```python
from build123d import *

# Parameters (mm, degrees)
SKETCH1_W           = 12.7
SKETCH1_H           = 31.75
SKETCH1_R           = 1.5875
BOSS_EXTRUDE2_DEPTH = 6.35
SKETCH1_5_R         = 1.27
CUT_EXTRUDE2_DEPTH  = 19.238986403
FILLET2_R           = 3.175
FILLET3_R           = 0.635


with BuildPart() as part:
    # Sketch1 → Boss-Extrude2 (new body)
    with BuildSketch(Plane(origin=(0, 0, 0), x_dir=(1, 0, 0), z_dir=(0, 1, 0))):
        Rectangle(SKETCH1_W, SKETCH1_H)
        with Locations(Location((0, -7.9375, 0), (0, 0, 270))):
            Circle(SKETCH1_R, mode=Mode.SUBTRACT)
    extrude(amount=BOSS_EXTRUDE2_DEPTH)

    # Sketch1_5 → Cut-Extrude2 (cut, through all)
    with BuildSketch(Plane(origin=(0, 0, 0), x_dir=(1, 0, 0), z_dir=(0, 1, 0))):
        with BuildLine():
            Line((-6.35, 3.701051224), (-6.35, -1.213547665))
            Line((-6.35, -1.213547665), (0.969401523, 7.434536298))
            ThreePointArc((0.969401523, 7.434536298), (-0.859985471, 7.320481413), (-0.898025612, 9.153025612))
            Line((-0.898025612, 9.153025612), (-6.35, 3.701051224))
        make_face()
        with Locations((0, 8.255)):
            Circle(SKETCH1_5_R)
    extrude(amount=CUT_EXTRUDE2_DEPTH, mode=Mode.SUBTRACT)

    # Fillet2
    fillet2_edges = [part.edges().sort_by_distance(p)[0] for p in [
        (6.35, 3.175, -15.875),
        (-6.35, 3.175, -15.875),
        (-6.35, 3.175, 15.875),
        (6.35, 3.175, 15.875),
    ]]
    fillet(fillet2_edges, radius=FILLET2_R)

    # Fillet3
    fillet3_edges = [part.edges().sort_by_distance(p)[0] for p in [
        (-6.35, 3.175, 1.213547665),
        (-6.35, 3.175, -3.701051224),
    ]]
    fillet(fillet3_edges, radius=FILLET3_R)


solid = part.part
```
Work out the finished part from the listing and answer in its coordinate system (mm). A direction names the side the tool comes from. Give positions to 0.01 mm unless a question says otherwise; leave off trailing zeros. Loops run counter-clockwise (first coordinate to the right, second up) from the corner with the lowest first, then second, coordinate; pieces in that order, holes last. Notation, with made-up numbers: (68.25, 86.25) -> (112.25, 86.25) arc R35 cw to (112.25, 122.25) -> close; hole circle Ø7 at (14, 30). An arc over 180 degrees is marked (long way). One line per question, with ' | ' between items. Start each with the question number.
1) Section B-B, the plane x = 0 is taken. Determine the outline of the cut face in (y, z) (3 decimals).
2) Section D-D, the plane x = 5 is taken. Determine the outline of the cut face in (y, z).
3) Determine the mould class of faces 3 (the face through (5.395, 3.219, -14.97)), 4 (the face through (-6.35, 3, 7)), 5 (the face through (-3.05, 3.13, -7)) for opening direction Z: +Z half, -Z half, draft (parallel to the pull), parting line (faces both ways), or undercut.
4) Section C-C, the plane z = -6 is taken. Determine the outline of the cut face in (x, y), then the cut area to 3 significant figures.
5) For faces 1 (the face through (-5.948, 3.219, -4.643)), 2 (the face through (5.395, 3.219, 14.97)), determine the directions among +Z, -Z, +X, -X, +Y, -Y from which every point of the face is accessible in a straight line to the end or side of a thin tool.
6) Straight lines are drawn through the part: L1, parallel to Z at x = -4.5, y = 1; L2, parallel to Z at x = -4, y = 3; L3, parallel to Z at x = -1, y = 4.25 (3 decimals). For each, find the intervals that lie inside material, in ascending order.
Resolved:
1) outline: (0, -15.875) -> (6.35, -15.875) -> (6.35, -9.525) -> (0, -9.525) -> close; (0, -6.289) -> (6.35, -6.289) -> (6.35, 6.35) -> (0, 6.35) -> close; (0, 9.525) -> (6.35, 9.525) -> (6.35, 15.875) -> (0, 15.875) -> close
2) outline: (0, -15.3) -> (6.35, -15.3) -> (6.35, 15.3) -> (0, 15.3) -> close
3) face 3: -Z half | face 4: draft | face 5: undercut
4) outline: (-6.35, 0) -> (-4.05, 0) -> (-4.05, 6.35) -> (-6.35, 6.35) -> close; (-0.24, 0) -> (6.35, 0) -> (6.35, 6.35) -> (-0.24, 6.35) -> close | area: 56.5 mm2
5) face 1: +Y, -Y | face 2: +Z, +X, +Y, -Y
6) L1: -15.59 to -5.55, -0.97 to 15.59 | L2: -15.77 to -6.05, -1.56 to 15.77 | L3: -15.875 to -9.051, -5.108 to 6.705, 9.17 to 15.875
